Read the model definition and answer for the solid it produces. Units are mm, in the model's axes. A direction names the side the tool comes from. Round coordinates to 2 decimals unless told otherwise and drop trailing zeros. Loops run counter-clockwise (first coordinate to the right, second up) from the corner with the lowest first, then second, coordinate; pieces in that order, holes last. Notation, with made-up numbers: M 69,14.5 L 84,14.5 A18 cw 84,26.5 Z; hole C -5,-16.75 d6. An arc over 180 degrees is marked long. Write each question's results on one line, items separated by ' | '.
Autodesk Inventor part; units mm, degrees
ref_plane "YZ Plane" through (0, 0, 0) normal (1, 0, 0) x (0, 1, 0)
ref_plane "XZ Plane" through (0, 0, 0) normal (0, 1, 0) x (-1, 0, 0)
ref_plane "XY Plane" through (0, 0, 0) normal (0, 0, 1) x (1, 0, 0)
sketch "Szkic1" plane through (0, 0, 0) normal (0, 0, 1) x (1, 0, 0)
  line L0 (-12.5, -10) -> (12.5, -10)
  line L1 (12.5, -10) -> (12.5, 10)
  line L2 (12.5, 10) -> (-12.5, 10)
  line L3 (-12.5, 10) -> (-12.5, -10)
  line L4 (-12.5, -10) -> (12.5, 10) construction
  line L5 (12.5, -10) -> (-12.5, 10) construction
  point P0 (0, 0)
  dimension "d0" = 25
  dimension "d1" = 20
extrude "Wyciągnięcie proste1" add sketch "Szkic1" along normal blind 3
sketch "Szkic2" plane through (0, 0, 3) normal (0, 0, 1) x (1, 0, 0)
  line L0 (1.25, -10) -> (4.25, -10)
  line L1 (4.25, -10) -> (4.25, 10)
  line L2 (4.25, 10) -> (1.25, 10)
  line L3 (1.25, 10) -> (1.25, -10)
  line L4 (1.25, -10) -> (4.25, 10) construction
  line L5 (4.25, -10) -> (1.25, 10) construction
  line L6 (-12.5, -10) -> (12.5, -10)
  line L7 (12.5, 10) -> (-12.5, 10)
  line L8 (0, 10) -> (0, -10) construction
  line L9 (-1.25, -10) -> (-4.25, -10)
  line L10 (-4.25, -10) -> (-4.25, 10)
  line L11 (-4.25, 10) -> (-1.25, 10)
  line L12 (-1.25, 10) -> (-1.25, -10)
  line L13 (-1.25, -10) -> (-4.25, 10) construction
  line L14 (-4.25, -10) -> (-1.25, 10) construction
  point P0 (0, 0)
  point P1 (2.75, 0)
  point P2 (-2.75, 0)
  dimension "d4" = 3
  dimension "d5" = 20
  dimension "d6" = 2.75
  dimension "d7" = 10
extrude "Wyciągnięcie proste2" add sketch "Szkic2" along normal blind 20 contours L3 L2 L1 L0 | L6 L10 L7 L12
sketch "Szkic3" plane through (4.25, -10, 3) normal (1, 0, 0) x (0, 0, -1)
  line L0 (-20, 0) -> (-20, 20)
  line L1 (0, 20) -> (-20, 20)
  point P0 (3, 10)
  point P1 (-17, 10)
  dimension "d10" = 3
  dimension "d11" = 10
hole "Otwór1" at (4.25, 0, 20) direction (-1, 0, 0) diameter 3 end through all
fillet "Zaokrąglenie1" radius 5 4 edges at (2.75, -10, 23) (-2.75, -10, 23) (-2.75, 10, 23) (2.75, 10, 23)
fillet "Zaokrąglenie2" radius 3 4 edges at (12.5, 10, 1.5) (12.5, -10, 1.5) (-12.5, -10, 1.5) (-12.5, 10, 1.5)
sketch "Szkic4" plane through (0, 0, 3) normal (0, 0, 1) x (1, 0, 0)
  line L0 (-12.5, 7) -> (-12.5, -7)
  line L1 (-9.5, -10) -> (-4.25, -10)
  line L2 (-1.25, -10) -> (1.25, -10)
  line L3 (0, -10) -> (0, 10) construction
  line L4 (1.25, 10) -> (-1.25, 10)
  line L5 (12.5, -7) -> (12.5, 7)
  line L6 (12.5, 0) -> (-12.5, 0) construction
  point P0 (0, 0)
  point P1 (-8.375, -5)
  point P2 (8.375, -5)
  point P3 (-8.375, 5)
  point P4 (8.375, 5)
  dimension "d21" = 4.125
  dimension "d22" = 5
hole "Otwór2" at (-8.375, -5, 3) at (8.375, -5, 3) at (8.375, 5, 3) at (-8.375, 5, 3) direction (0, 0, -1) diameter 3 end through all
properties part number "pleksi_mocowanie"
1. Find section D-D, the plane x = -8. Give the vertices of the cut face in (y, z), then the cut area to 3 significant figures.
Completed:
outline: M -10,0 L -6.45,0 L -6.45,3 L -10,3 Z; M -3.55,0 L 3.55,0 L 3.55,3 L -3.55,3 Z; M 6.45,0 L 10,0 L 10,3 L 6.45,3 Z | area: 42.6 mm2
2. Determine the mould class of faces 4 (the face through (-11.6, 9.14, 1.52)), 5 (the face through (0, 0, 3)), 6 (the face through (-2.77, -0.07, 21.5)), 7 (the face through (2.73, -0.07, 21.5)) for opening direction Z: released by +Z, released by -Z, zero draft, split by the parting line, or undercut.
Completed:
face 4: zero draft | face 5: released by +Z | face 6: undercut | face 7: undercut
3. Find section B-B, the plane z = 13.5. Give the vertices of the cut face in (x, y), then the cut area to 3 significant figures.
Completed:
outline: M -4.25,-10 L -1.25,-10 L -1.25,10 L -4.25,10 Z; M 1.25,-10 L 4.25,-10 L 4.25,10 L 1.25,10 Z | area: 120 mm2
4. Find section A-A, the plane y = 0. Give the vertices of the cut face in (x, z), then the cut area to 3 significant figures.
Completed:
outline: M -12.5,0 L 12.5,0 L 12.5,3 L 4.25,3 L 4.25,18.5 L 1.25,18.5 L 1.25,3 L -1.25,3 L -1.25,18.5 L -4.25,18.5 L -4.25,3 L -12.5,3 Z; M -4.25,21.5 L -1.25,21.5 L -1.25,23 L -4.25,23 Z; M 1.25,21.5 L 4.25,21.5 L 4.25,23 L 1.25,23 Z | area: 177 mm2
5. Find section C-C, the plane z = 20. Give the vertices of the cut face in (x, y), then the cut area to 3 significant figures.
Completed:
outline: M -4.25,-9.58 L -1.25,-9.58 L -1.25,-1.5 L -4.25,-1.5 Z; M -4.25,1.5 L -1.25,1.5 L -1.25,9.58 L -4.25,9.58 Z; M 1.25,-9.58 L 4.25,-9.58 L 4.25,-1.5 L 1.25,-1.5 Z; M 1.25,1.5 L 4.25,1.5 L 4.25,9.58 L 1.25,9.58 Z | area: 97.0 mm2
6. Given P1, Ø6, axis at y = 3.5, z = 13.5, coming from the +X side; P2, Ø2.5, axis at y = 0, z = 20, coming from the -X side; P3, Ø12, axis at y = -7.5, z = 9.5, coming from the -X side; P4, Ø5, axis at x = -8.375, y = -5, coming from the +Z side, each flat-ended and moving along its own axis, determine where each tip first touches the part or whether it passes through.
Completed:
P1: stops at x = 4.25 | P2: passes through | P3: stops at x = -4.25 | P4: stops at z = 3
7. Which of the six approach directions +Z, -Z, +X, -X, +Y, -Y give full straight-line access (tool end or side, diameter ignored) to faces 1 (the face through (-8, 0, 3)), 2 (the face through (-1.25, 0, 13)), 3 (the face through (11.64, 9.1, 1.52))?
Completed:
face 1: +Z, -X, +Y, -Y | face 2: +Z, +Y, -Y | face 3: +Z, -Z, +X, +Y
8. Find the intervals of material crossed by L1, parallel to Z at x = -3.6, y = 0; L2, parallel to X at y = 5, z = 2.45 (3 decimals); L3, parallel to X at y = -3, z = 21.5, in increasing order.
Completed:
L1: z = 0 to 18.5, 21.5 to 23 | L2: x = -12.5 to -9.875, -6.875 to 6.875, 9.875 to 12.5 | L3: x = -4.25 to -1.25, 1.25 to 4.25
